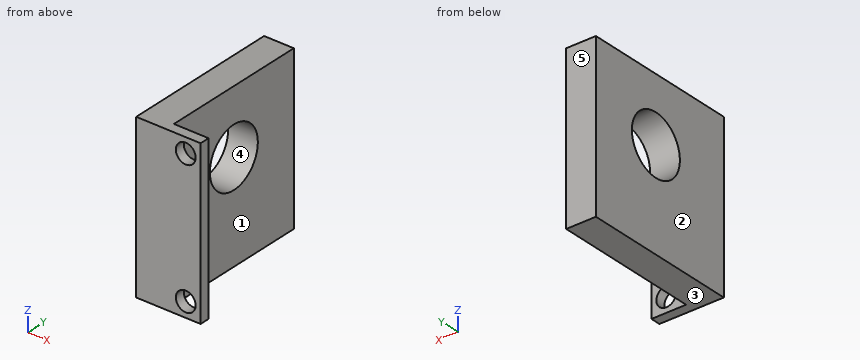
from build123d import *

# Parameters (mm, degrees)
BOSS_EXTRUDE1_DEPTH = 33
CUT_EXTRUDE1_REACH  = 48.497
SKETCH2_R           = 6
CUT_EXTRUDE2_REACH  = 48.454
SKETCH3_R           = 2


with BuildPart() as part:
    # Sketch1 → Boss-Extrude1 (new body)
    with BuildSketch(Plane.XY):
        Polygon((0, 0), (0, 32), (6, 32), (6, 2), (13, 2), (13, 0), align=None)
    extrude(amount=BOSS_EXTRUDE1_DEPTH)

    # Sketch2 → Cut-Extrude1 (cut, up to next)
    with BuildSketch(Plane(origin=(6, 0, 0), x_dir=(0, 0, -1), z_dir=(1, 0, 0)), mode=Mode.PRIVATE) as cut_extrude1_sk1:
        with Locations(Location((-20, 17, 0), (0, 0, 90))):
            Circle(SKETCH2_R)
    cut_extrude1_tool1 = extrude(cut_extrude1_sk1.sketch, amount=-CUT_EXTRUDE1_REACH, mode=Mode.PRIVATE) & part.part
    add(cut_extrude1_tool1.solids().sort_by_distance((6, 17, 20))[0], mode=Mode.SUBTRACT)

    # Sketch3 → Cut-Extrude2 (cut, up to next)
    with BuildSketch(Plane(origin=(0, 2, 0), x_dir=(1, 0, 0), z_dir=(0, 1, 0)), mode=Mode.PRIVATE) as cut_extrude2_sk1:
        with Locations(Location((10, -3, 0), (0, 0, 180))):
            Circle(SKETCH3_R)
    cut_extrude2_tool1 = extrude(cut_extrude2_sk1.sketch, amount=-CUT_EXTRUDE2_REACH, mode=Mode.PRIVATE) & part.part
    # Sketch3 → Cut-Extrude2 (cut, up to next)
    with BuildSketch(Plane(origin=(0, 2, 0), x_dir=(1, 0, 0), z_dir=(0, 1, 0)), mode=Mode.PRIVATE) as cut_extrude2_sk2:
        with Locations(Location((10, -30, 0), (0, 0, 180))):
            Circle(SKETCH3_R)
    cut_extrude2_tool2 = extrude(cut_extrude2_sk2.sketch, amount=-CUT_EXTRUDE2_REACH, mode=Mode.PRIVATE) & part.part
    add(cut_extrude2_tool1.solids().sort_by_distance((10, 2, 3))[0], mode=Mode.SUBTRACT)
    add(cut_extrude2_tool2.solids().sort_by_distance((10, 2, 30))[0], mode=Mode.SUBTRACT)


solid = part.part
Design review of the part built by this model. Coordinates are the model's own, in mm. Face numbers are marked on the shaded views. A direction names the side the tool comes from. Round coordinates to 2 decimals unless told otherwise and drop trailing zeros. Write each loop counter-clockwise with the first axis right and the second up, starting at its lowest first coordinate (ties: lowest second). Pieces come first, ordered by that corner, then holes.
Item 1: Consider section D-D on z = 13. Give the boundary of the cut face in (x, y).
Item 2: Draft analysis for pull direction Z (two halves, no side actions). For the marked faces 3, 4 and 5, state which applies: released by +Z, released by -Z, zero draft, split by the parting line, or undercut.
Item 3: Consider section A-A on z = 3. Give the boundary of the cut face in (x, y), and give its area (3 significant figures).
Item 4: Consider section C-C on y = 17. Give the boundary of the cut face in (x, z).
Item 5: For pin 1 Ø5 at (x, z) = (10, 30) entering from +Y; pin 2 Ø9 at (y, z) = (12.5, 9) entering from +X, all flat-tipped, find the tip position at first contact; note any pin that passes through.
Item 6: Wall thickness on L1, parallel to Z at x = 10, y = 0.6; L2, parallel to Z at x = 4.5, y = 17; L3, parallel to Y at x = 0.75, z = 22: over which ranges is each line inside the solid? List them lowest first.
Item 7: For the marked faces 1 and 2, list the 3-axis set-ups (+Z, -Z, +X, -X, +Y, -Y) from which the entire face can be reached by the end or side of a thin tool; tool diameter is ignored.
Item 8: Consider section B-B on x = 10. Give the boundary of the cut face in (y, z), and give its area (3 significant figures).
Check values:
1. outline: (0, 0) - (13, 0) - (13, 2) - (6, 2) - (6, 32) - (0, 32) - close
2. face 3: released by -Z
2. face 4: undercut
2. face 5: zero draft
3. outline: (0, 0) - (8, 0) - (8, 2) - (6, 2) - (6, 32) - (0, 32) - close; (12, 0) - (13, 0) - (13, 2) - (12, 2) - close
3. area: 198 mm2
4. outline: (0, 0) - (6, 0) - (6, 14) - (0, 14) - close; (0, 26) - (6, 26) - (6, 33) - (0, 33) - close
5. pin 1: stops at y = 2
5. pin 2: stops at x = 6
6. L1: z = 0 to 1, 5 to 28, 32 to 33
6. L2: z = 0 to 14, 26 to 33
6. L3: y = 0 to 11.34, 22.66 to 32
7. face 1: +Z, -Z, +X, +Y
7. face 2: +Z, -Z, -X, +Y, -Y
8. outline: (0, 0) - (2, 0) - (2, 1) - (0, 1) - close; (0, 5) - (2, 5) - (2, 28) - (0, 28) - close; (0, 32) - (2, 32) - (2, 33) - (0, 33) - close
8. area: 50.0 mm2
